from build123d import *

# Parameters (mm, degrees)
F0_W     = 75
F0_H     = 75
F1_DEPTH = 10
F3_DEPTH = 25
F4_DEPTH = 10


with BuildPart() as f1:
    # F0 (on Top) → F1 (new body)
    with BuildSketch(Plane.XY):
        Rectangle(F0_W, F0_H)
    extrude(amount=F1_DEPTH)

    # F2 (on face) → F3 (join)
    with BuildSketch(Plane.XY.offset(10)):
        with BuildLine():
            ThreePointArc((0, 6), (-4.242641, -4.242641), (6, 0))
            ThreePointArc((6, 0), (4.242641, 4.242641), (0, 6))
        make_face()
    extrude(amount=F3_DEPTH)

    # F2 (on face) → F4 (cut)
    with BuildSketch(Plane.XY.offset(10)):
        with BuildLine():
            ThreePointArc((2.5, 15), (-1.767767, 16.767767), (0, 12.5))
            ThreePointArc((0, 12.5), (1.767767, 13.232233), (2.5, 15))
        make_face()
    extrude(amount=-F4_DEPTH, mode=Mode.SUBTRACT)


solid = f1.part
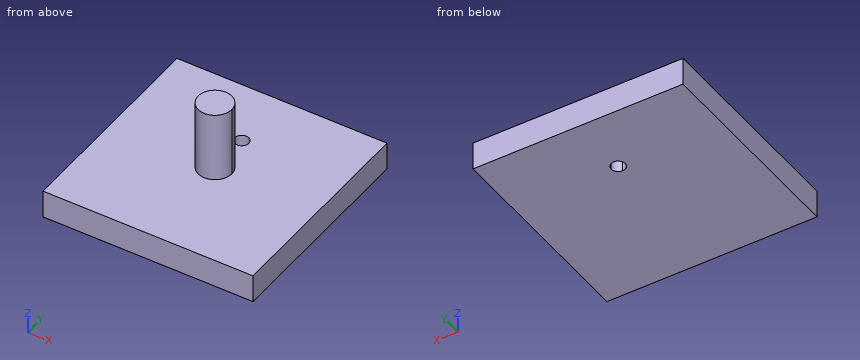
Verification items for the finished model (mm, model axes). Coordinates: 2 decimals unless noted, no trailing zeros. Order: outer loops, then holes, each group sorted by start corner. A loop starts at its lowest first (then second) coordinate and runs counter-clockwise, first axis right, second up. Notation, with made-up numbers: M 24,-13.5 L 49,-13.5 A26 cw 49,21.5 Z; hole C -20.75,-24.5 d5. An arc over 180 degrees is marked long. One line per item, written item: value. Start each with the question number.
Item 1: Sectioned sample at D-D on x = 3.5. Record the cut outline in (y, z).
Item 2: Depth check by flat-ended pin: P1, Ø6, axis at x = -2.5, y = 29.5, coming from the +Z side; P2, Ø8, axis at x = 12.5, z = 31, coming from the -Y side. Enter the tip coordinate at first touch or a pass-through.
Item 3: Sectioned sample at C-C on z = 18.5. Record the cut outline in (x, y), then the cut area to 3 significant figures.
Item 4: Sectioned sample at A-A on y = 16. Record the cut outline in (x, z).
Item 5: Thickness scan on probe 1 along Y at (x, z) = (0, 7); probe 2 along X at (y, z) = (15, 5.5); probe 3 along Z at (x, y) = (-15.5, 11). Record the ranges inside material, lowest first.
Item 6: Sectioned sample at B-B on y = -8. Record the cut outline in (x, z), then the cut area to 3 significant figures.
Calculated:
1. outline: M -37.5,0 L 37.5,0 L 37.5,10 L 4.87,10 L 4.87,35 L -4.87,35 L -4.87,10 L -37.5,10 Z
2. P1: z = 10
2. P2: through
3. outline: M 0,6 A6 ccw long 6,0 A6 ccw Z
3. area: 113 mm^2
4. outline: M -37.5,0 L -2.29,0 L -2.29,10 L -37.5,10 Z; M 2.29,0 L 37.5,0 L 37.5,10 L 2.29,10 Z
5. probe 1: -37.5 to 12.5, 17.5 to 37.5
5. probe 2: -37.5 to -2.5, 2.5 to 37.5
5. probe 3: 0 to 10
6. outline: M -37.5,0 L 37.5,0 L 37.5,10 L -37.5,10 Z
6. area: 750 mm^2
